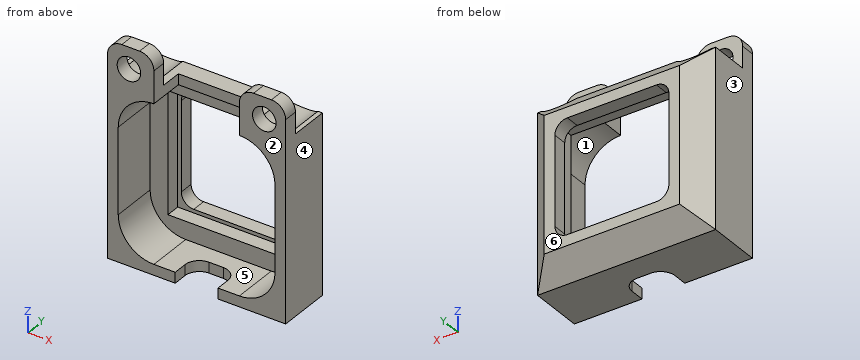
from build123d import *

# Parameters (mm, degrees)
SZKIC1_W                    = 25
SZKIC1_H                    = 25
DODANIE_WYCI_GNI_CIE1_DEPTH = 2
SZKIC2_W                    = 25
SZKIC2_H                    = 25
SZKIC2_W_2                  = 17
SZKIC2_H_2                  = 17
DODANIE_WYCI_GNI_CIE2_DEPTH = 2
SZKIC3_W                    = 25
SZKIC3_H                    = 25
SZKIC3_W_2                  = 22
SZKIC3_H_2                  = 22
DODANIE_WYCI_GNI_CIE3_DEPTH = 6.5
SZKIC4_W                    = 12
SZKIC4_H                    = 5
WYTNIJ_WYCI_GNI_CIE1_DEPTH  = 1.5
SFAZOWANIE1_SIZE            = 3
SZKIC5_W                    = 6.5
SZKIC5_H                    = 5
DODANIE_WYCI_GNI_CIE4_DEPTH = 2
SZKIC8_R                    = 1.65
WYTNIJ_WYCI_GNI_CIE3_DEPTH  = 24.932195888
ZAOKR_GLENIE1_R             = 2
WYTNIJ_WYCI_GNI_CIE4_START  = -2
SZKIC9_R                    = 3.1
WYTNIJ_WYCI_GNI_CIE4_DEPTH  = 22.932195888
ZAOKR_GLENIE1_OF_LUSTRO1_R  = 2
SZKIC6_W                    = 6
SZKIC6_H                    = 4
WYTNIJ_WYCI_GNI_CIE2_DEPTH  = 10
ZAOKR_GLENIE4_R             = 2
ZAOKR_GLENIE5_R             = 5


with BuildPart() as part:
    # Szkic1 → Dodanie-wyciągnięcie1 (new body)
    with BuildSketch(Plane(origin=(0, 0, 0), x_dir=(1, 0, 0), z_dir=(0, 1, 0))):
        Rectangle(SZKIC1_W, SZKIC1_H)
        with BuildLine():
            Line((-6.25, 8), (6.25, 8))
            ThreePointArc((6.25, 8), (7.487436867, 7.487436867), (8, 6.25))
            Line((8, 6.25), (8, -6.25))
            ThreePointArc((8, -6.25), (7.487436867, -7.487436867), (6.25, -8))
            Line((6.25, -8), (-6.25, -8))
            ThreePointArc((-6.25, -8), (-7.487436867, -7.487436867), (-8, -6.25))
            Line((-8, -6.25), (-8, 6.25))
            ThreePointArc((-8, 6.25), (-7.487436867, 7.487436867), (-6.25, 8))
        make_face(mode=Mode.SUBTRACT)
    extrude(amount=-DODANIE_WYCI_GNI_CIE1_DEPTH)

    # Szkic2 → Dodanie-wyciągnięcie2 (add)
    with BuildSketch(Plane.XZ.offset(2)):
        Rectangle(SZKIC2_W, SZKIC2_H)
        Rectangle(SZKIC2_W_2, SZKIC2_H_2, mode=Mode.SUBTRACT)
    extrude(amount=DODANIE_WYCI_GNI_CIE2_DEPTH)

    # Szkic3 → Dodanie-wyciągnięcie3 (add)
    with BuildSketch(Plane.XZ.offset(4)):
        Rectangle(SZKIC3_W, SZKIC3_H)
        Rectangle(SZKIC3_W_2, SZKIC3_H_2, mode=Mode.SUBTRACT)
    extrude(amount=DODANIE_WYCI_GNI_CIE3_DEPTH)

    # Szkic4 → Wytnij-wyciągnięcie1 (cut)
    with BuildSketch(Plane.XY.offset(12.5)):
        with Locations((0, -8)):
            Rectangle(SZKIC4_W, SZKIC4_H)
    extrude(amount=-WYTNIJ_WYCI_GNI_CIE1_DEPTH, mode=Mode.SUBTRACT)

    # Sfazowanie1
    sfazowanie1_edges = [part.edges().sort_by_distance(p)[0] for p in [
        (0, 0, 12.5),
        (-12.5, 0, 0),
        (0, 0, -12.5),
        (12.5, 0, 0),
    ]]
    chamfer(sfazowanie1_edges, length=SFAZOWANIE1_SIZE)

    # Szkic5 → Dodanie-wyciągnięcie4 (add)
    with BuildSketch(Plane.XZ.offset(10.5)):
        with Locations((-9.25, 15)):
            Rectangle(SZKIC5_W, SZKIC5_H)
    dodanie_wyci_gni_cie4 = extrude(amount=-DODANIE_WYCI_GNI_CIE4_DEPTH)

    # Szkic8 → Wytnij-wyciągnięcie3 (cut, through all)
    with BuildSketch(Plane.XZ.offset(10.5)):
        with Locations(Location((-9.5, 14.5, 0), (0, 0, 270))):
            Circle(SZKIC8_R)
    wytnij_wyci_gni_cie3 = extrude(amount=-WYTNIJ_WYCI_GNI_CIE3_DEPTH, mode=Mode.SUBTRACT)

    # Zaokrąglenie1
    zaokr_glenie1_edges = [part.edges().sort_by_distance(p)[0] for p in [
        (-12.5, -9.5, 17.5),
        (-6, -9.5, 17.5),
    ]]
    fillet(zaokr_glenie1_edges, radius=ZAOKR_GLENIE1_R)

    # Szkic9 → Wytnij-wyciągnięcie4 (cut, through all)
    with BuildSketch(Plane.XZ.offset(10.5).offset(WYTNIJ_WYCI_GNI_CIE4_START)):
        with Locations((-9.5, 14.5)):
            Circle(SZKIC9_R)
    wytnij_wyci_gni_cie4 = extrude(amount=-WYTNIJ_WYCI_GNI_CIE4_DEPTH, mode=Mode.SUBTRACT)

    # Lustro1: Dodanie-wyciągnięcie4, Wytnij-wyciągnięcie3, Wytnij-wyciągnięcie4 across plane
    add(dodanie_wyci_gni_cie4.mirror(Plane(origin=(0, 0, 0), x_dir=(0, 0, 1), z_dir=(1, 0, 0))))
    add(wytnij_wyci_gni_cie3.mirror(Plane(origin=(0, 0, 0), x_dir=(0, 0, 1), z_dir=(1, 0, 0))), mode=Mode.SUBTRACT)
    add(wytnij_wyci_gni_cie4.mirror(Plane(origin=(0, 0, 0), x_dir=(0, 0, 1), z_dir=(1, 0, 0))), mode=Mode.SUBTRACT)

    # Zaokrąglenie1 of Lustro1
    zaokr_glenie1_of_lustro1_edges = [part.edges().sort_by_distance(p)[0] for p in [
        (12.5, -9.5, 17.5),
        (6, -9.5, 17.5),
    ]]
    fillet(zaokr_glenie1_of_lustro1_edges, radius=ZAOKR_GLENIE1_OF_LUSTRO1_R)

    # Szkic6 → Wytnij-wyciągnięcie2 (cut)
    with BuildSketch(Plane(origin=(0, 0, -12.5), x_dir=(-1, 0, 0), z_dir=(0, 0, -1))):
        with Locations((0, -8.5)):
            Rectangle(SZKIC6_W, SZKIC6_H)
    extrude(amount=-WYTNIJ_WYCI_GNI_CIE2_DEPTH, mode=Mode.SUBTRACT)

    # Zaokrąglenie4
    zaokr_glenie4_edges = [part.edges().sort_by_distance(p)[0] for p in [
        (3, -6.5, -11.75),
        (-3, -6.5, -11.75),
    ]]
    fillet(zaokr_glenie4_edges, radius=ZAOKR_GLENIE4_R)

    # Zaokrąglenie5
    zaokr_glenie5_edges = [part.edges().sort_by_distance(p)[0] for p in [
        (11, -7.25, -11),
        (-11, -7.25, -11),
        (-11, -7.25, 11),
        (11, -7.25, 11),
    ]]
    fillet(zaokr_glenie5_edges, radius=ZAOKR_GLENIE5_R)


solid = part.part
The model under review builds one solid part; all positions refer to its coordinate system, in mm. Face numbers are marked on the shaded views. A direction names the side the tool comes from. Give positions to 0.01 mm unless a question says otherwise; leave off trailing zeros. Write each loop counter-clockwise with the first axis right and the second up, starting at its lowest first coordinate (ties: lowest second). Pieces come first, ordered by that corner, then holes.
1. Add section C-C, the plane z = 14.5. Write out the cut boundary in (x, y), plus the area to 3 significant figures.
2. Add section D-D, the plane y = -9.5. Write out the cut boundary in (x, z), plus the area to 3 significant figures.
3. Add section B-B, the plane y = -4.5. Write out the cut boundary in (x, z).
4. Draft analysis for pull direction X (two halves, no side actions). For the marked faces 3, 4, 5 and 6, state which applies: +X half, -X half, draft (parallel to the pull), parting line (faces both ways), or undercut.
5. Wall thickness on L1, parallel to X at y = -9.8, z = 14.5; L2, parallel to X at y = -9.5, z = 11.25; L3, parallel to X at y = -6.5, z = 5.75: over which ranges is each line inside the solid? List them lowest first.
6. Add section A-A, the plane z = 1. Write out the cut boundary in (x, y).
7. For P1, Ø1.2, axis at x = -3, z = 11.5, coming from the -Y side; P2, Ø2, axis at x = -4, y = -3.5, coming from the +Z side; P3, Ø0.6, axis at y = -0.5, z = 2, coming from the -X side, all flat-tipped, find the tip position at first contact; note any pin that passes through.
8. Tool access review of the marked faces 1 and 2: name each direction out of +Z, -Z, +X, -X, +Y, -Y from which nothing blocks a thin tool from reaching the whole face with its end or side.
Worked answers:
1. outline: (-12.5, -10.5) - (-11.15, -10.5) - (-11.15, -8.5) - (-12.5, -8.5) - close; (-7.85, -10.5) - (-6, -10.5) - (-6, -8.5) - (-7.85, -8.5) - close; (6, -10.5) - (7.85, -10.5) - (7.85, -8.5) - (6, -8.5) - close; (11.15, -10.5) - (12.5, -10.5) - (12.5, -8.5) - (11.15, -8.5) - close
1. area: 12.8 mm2
2. outline: (-12.5, -12.5) - (-3, -12.5) - (-3, -11) - (-6, -11) arc R5 cw to (-11, -6) - (-11, 6) arc R5 cw to (-6, 11) - (-6, 15.5) arc R2 ccw to (-8, 17.5) - (-10.5, 17.5) arc R2 ccw to (-12.5, 15.5) - close; (3, -12.5) - (12.5, -12.5) - (12.5, 15.5) arc R2 ccw to (10.5, 17.5) - (8, 17.5) arc R2 ccw to (6, 15.5) - (6, 11) arc R5 cw to (11, 6) - (11, -6) arc R5 cw to (6, -11) - (3, -11) - close; hole circle Ø3.3 at (-9.5, 14.5); hole circle Ø3.3 at (9.5, 14.5)
2. area: 180 mm2
3. outline: (-12.5, -12.5) - (12.5, -12.5) - (12.5, 12.5) - (11.87, 12.5) arc R3.1 cw to (7.13, 12.5) - (-7.13, 12.5) arc R3.1 cw to (-11.87, 12.5) - (-12.5, 12.5) - close; hole (-11, -6) arc R5 ccw to (-6, -11) - (6, -11) arc R5 ccw to (11, -6) - (11, 6) arc R5 ccw to (6, 11) - (-6, 11) arc R5 ccw to (-11, 6) - close
4. face 3: -X half
4. face 4: +X half
4. face 5: undercut
4. face 6: draft
5. L1: x = -12.5 to -11.15, -7.85 to -6, 6 to 7.85, 11.15 to 12.5
5. L2: x = -12.5 to -6, 6 to 12.5
5. L3: x = -12.5 to -11, 11 to 12.5
6. outline: (-12.5, -10.5) - (-11, -10.5) - (-11, -4) - (-8.5, -4) - (-8.5, -2) - (-8, -2) - (-8, 0) - (-9.5, 0) - (-12.5, -3) - close; (8, -2) - (8.5, -2) - (8.5, -4) - (11, -4) - (11, -10.5) - (12.5, -10.5) - (12.5, -3) - (9.5, 0) - (8, 0) - close
7. P1: stops at y = -5.5
7. P2: stops at z = 12.5
7. P3: stops at x = -10.3
8. face 1: -Y
8. face 2: +Z, -Z, +X, -X, -Y
